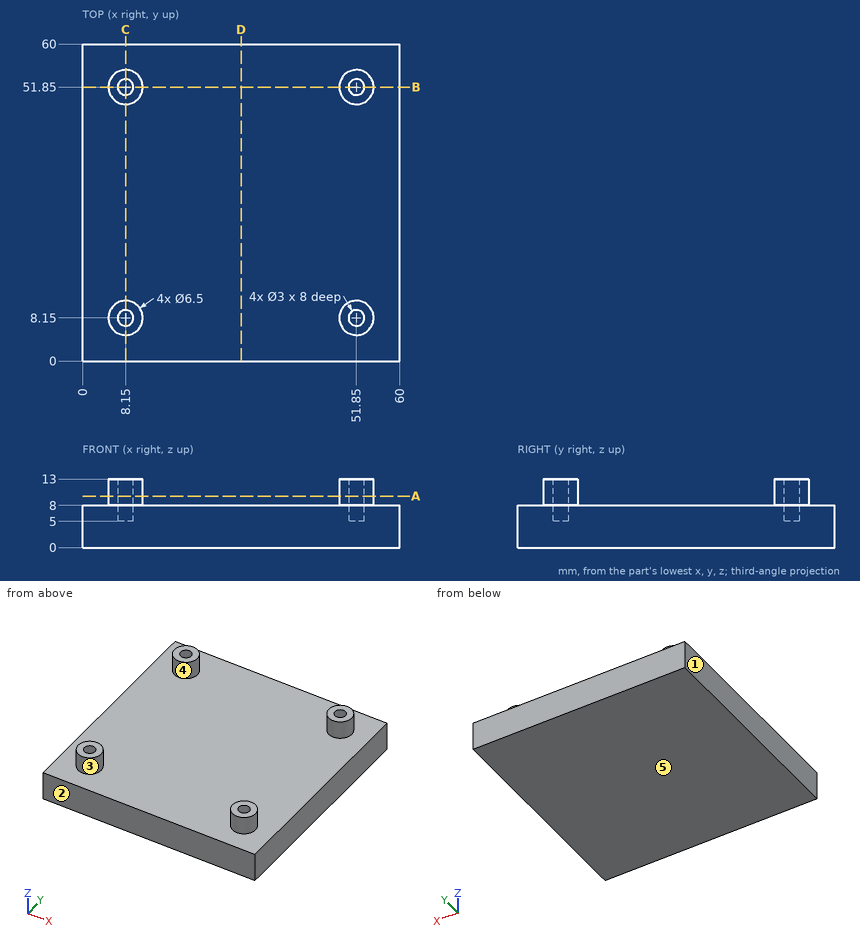
Could you check a few things on this drawing? It's one solid part, dimensions in mm from its lowest x, y, z. A direction names the side the tool comes from. Coordinates: 2 decimals unless noted, no trailing zeros. Order: outer loops, then holes, each group sorted by start corner. A loop starts at its lowest first (then second) coordinate and runs counter-clockwise, first axis right, second up. Notation, with made-up numbers: (20.5, 3) - (28.5, 3) arc R24 ccw to (28.5, 18) - close; hole circle Ø11 at (84, 62). An arc over 180 degrees is marked (long way). One line per question, with ' | ' between items.
(1) Will these pins go through, and if not, where does the flat tip stop? pin 1 (1.8 mm diameter, centred on x = 8.15, y = 51.85, fed in from +Z); pin 2 (4 mm diameter, centred on x = 36, y = 13.5, fed in from +Z); pin 3 (3 mm diameter, centred on y = 43.5, z = 11, fed in from +X).
Report:
pin 1: stops at z = 5 | pin 2: stops at z = 8 | pin 3: passes through
(2) Suppose I cut it at B-B on y = 51.85. List the corners of the cut face in (x, z) for me.
Report:
outline: (0, 0) - (60, 0) - (60, 8) - (55.1, 8) - (55.1, 13) - (53.35, 13) - (53.35, 5) - (50.35, 5) - (50.35, 13) - (48.6, 13) - (48.6, 8) - (11.4, 8) - (11.4, 13) - (9.65, 13) - (9.65, 5) - (6.65, 5) - (6.65, 13) - (4.9, 13) - (4.9, 8) - (0, 8) - close
(3) For the marked faces 4 and 5, which set-ups out of +Z, -Z, +X, -X, +Y, -Y let a thin tool reach every point of the face, with its end or its side?
Report:
face 4: +Z | face 5: -Z, +X, -X, +Y, -Y
(4) If we mould it in two halves opening along X, with no side actions, what happens to the marked faces 1, 2 and 3? For each: pulls with the +X half, pulls with the -X half, needs draft (parallel to the pull), parting line crosses it, or undercut.
Report:
face 1: pulls with the -X half | face 2: needs draft | face 3: undercut
(5) Suppose I cut it at D-D on x = 30. List the corners of the cut face in (y, z) for me.
Report:
outline: (0, 0) - (60, 0) - (60, 8) - (0, 8) - close
(6) If I drill on L1, parallel to Y at x = 51.85, z = 7; L2, parallel to Y at x = 51.85, z = 9; L3, parallel to Y at x = 7, z = 10.75, over which ranges is the centre line in solid material (lowest first)?
Report:
L1: y = 0 to 6.65, 9.65 to 50.35, 53.35 to 60 | L2: y = 4.9 to 6.65, 9.65 to 11.4, 48.6 to 50.35, 53.35 to 55.1 | L3: y = 5.11 to 7.19, 9.11 to 11.19, 48.81 to 50.89, 52.81 to 54.89
(7) Suppose I cut it at A-A on z = 9.75. List the corners of the cut face in (x, y) for me, and give its area (3 significant figures).
Report:
outline: circle Ø6.5 at (8.15, 8.15); circle Ø6.5 at (8.15, 51.85); circle Ø6.5 at (51.85, 8.15); circle Ø6.5 at (51.85, 51.85); hole circle Ø3 at (8.15, 8.15); hole circle Ø3 at (8.15, 51.85); hole circle Ø3 at (51.85, 8.15); hole circle Ø3 at (51.85, 51.85) | area: 104 mm2
